Read the model definition and answer for the solid it produces. Units are mm, in the model's axes. A direction names the side the tool comes from. Coordinates: 2 decimals unless noted, no trailing zeros. Write each loop counter-clockwise with the first axis right and the second up, starting at its lowest first coordinate (ties: lowest second). Pieces come first, ordered by that corner, then holes. Notation, with made-up numbers: (-3, 83.5) -> (20, 83.5) arc R20 ccw to (20, 107.5) -> close; hole circle Ø9 at (-18, 63.5). An arc over 180 degrees is marked (long way). Answer as a JSON object with one key per item and string values. Group by question number.
(1) Find section B-B (z = -11.5). Give the vertices of the cut face in (x, y), then the cut area to 3 significant figures.
(2) Find section C-C (x = 4). Give the vertices of the cut face in (y, z).
(3) Straight lines are drawn through the part: L1, parallel to Z at x = 8.75, y = 9.25; L2, parallel to Y at x = 1, z = 0; L3, parallel to X at y = 4.25, z = -11.5. For each, find the intervals that lie inside material, in ascending order.
(4) For a pull along Y with two mould halves and no side action, classify faces 1 (the face through (4, 4.2, 0)), 2 (the face through (9.699, 11.677, 5.714)), 3 (the face through (-5.74, 13.94, 5.71)), 4 (the face through (-3, 5, 0)) as +Y half, -Y half, draft (parallel to the pull), parting line (faces both ways), or undercut.
(5) Flat-ended cylindrical pins translate along their axes: P1, Ø1, axis at x = 3.5, y = 14.5, coming from the -Z side; P2, Ø1.8, axis at x = -4.5, z = 0, coming from the -Y side; P3, Ø0.5, axis at y = 3.5, z = 4, coming from the -X side. Find the tip coordinate at first contact, or state that the pin passes through.
(6) Find section A-A (x = 0). Give the vertices of the cut face in (y, z), then the cut area to 3 significant figures.
(7) Which of the six approach directions +Z, -Z, +X, -X, +Y, -Y give full straight-line access (tool end or side, diameter ignored) to faces 5 (the face through (-1.2, 3.1, 9.9)), 6 (the face through (-4, 4.2, 0)), 7 (the face through (0, 6.1, 14))?
(8) Find section D-D (z = -8). Give the vertices of the cut face in (x, y).
from build123d import *

# Parameters (mm, degrees)
BOSS_EXTRUDE1_DEPTH     = 16
SKETCH2_W               = 20
SKETCH2_H               = 11.997864578
BOSS_EXTRUDE2_DEPTH     = 12
CHAMFER1_SIZE           = 8
FILLET1_R               = 1
CUT_EXTRUDE1_DEPTH      = 27.145936587
CUT_EXTRUDE1_DEPTH_BACK = 27.145936587
SKETCH3_R               = 4
SKETCH4_R               = 2
CUT_EXTRUDE2_DEPTH      = 23.36067982


with BuildPart() as part:
    # Sketch1 → Boss-Extrude1 (new, symmetric)
    with BuildSketch(Plane.XY):
        Polygon((-3, 6.1), (3, 6.1), (3, 4.2), (5.3, 4.2), (5.3, 2.58), (2.8, 0), (-2.8, 0), (-5.3, 2.58), (-5.3, 4.2), (-3, 4.2), align=None)
    extrude(amount=BOSS_EXTRUDE1_DEPTH, both=True)

    # Sketch2 → Boss-Extrude2 (add)
    with BuildSketch(Plane(origin=(0, 6.1, 0), x_dir=(1, 0, 0), z_dir=(0, 1, 0))):
        Rectangle(SKETCH2_W, SKETCH2_H)
    extrude(amount=BOSS_EXTRUDE2_DEPTH)

    # Chamfer1
    chamfer1_edges = [part.edges().sort_by_distance(p)[0] for p in [
        (-10, 18.1, 0),
    ]]
    chamfer(chamfer1_edges, length=CHAMFER1_SIZE)

    # Fillet1
    fillet1_edges = [part.edges().sort_by_distance(p)[0] for p in [
        (0, 6.1, -5.998932289),
        (0, 6.1, 5.998932289),
        (-10, 6.1, 0),
        (-10, 8.1, 5.998932289),
        (-10, 8.1, -5.998932289),
        (10, 6.1, 0),
        (-6, 14.1, 5.998932289),
        (-6, 14.1, -5.998932289),
        (4, 18.1, -5.998932289),
        (4, 18.1, 5.998932289),
        (10, 12.1, -5.998932289),
        (10, 18.1, 0),
        (10, 12.1, 5.998932289),
        (-2, 18.1, 0),
        (-10, 10.1, 0),
    ]]
    fillet(fillet1_edges, radius=FILLET1_R)

    # Sketch3 → Cut-Extrude1 (cut, two sides: drawn at the far end of the back side and taken through both)
    with BuildSketch(Plane(origin=(0, 0, 0), x_dir=(0, 0, -1), z_dir=(1, 0, 0)).offset(-CUT_EXTRUDE1_DEPTH_BACK)):
        with Locations((0, 12.1)):
            Circle(SKETCH3_R)
    extrude(amount=CUT_EXTRUDE1_DEPTH + CUT_EXTRUDE1_DEPTH_BACK, mode=Mode.SUBTRACT)

    # Sketch4 → Cut-Extrude2 (cut, through all)
    with BuildSketch(Plane(origin=(0, 6.1, 0), x_dir=(1, 0, 0), z_dir=(0, 1, 0))):
        with Locations(Location((0, 11.5, 0), (0, 0, 270))):
            Circle(SKETCH4_R)
        with Locations(Location((0, -11.5, 0), (0, 0, 270))):
            Circle(SKETCH4_R)
    extrude(amount=-CUT_EXTRUDE2_DEPTH, mode=Mode.SUBTRACT)


solid = part.part
Results below:
{
 "1": {"outline": "(-5.3, 2.58) -> (-2.8, 0) -> (-2, 0) -> (-2, 6.1) -> (-3, 6.1) -> (-3, 4.2) -> (-5.3, 4.2) -> close; (2, 0) -> (2.8, 0) -> (5.3, 2.58) -> (5.3, 4.2) -> (3, 4.2) -> (3, 6.1) -> (2, 6.1) -> close", "area": "25.1 mm2"},
 "2": {"outline": "(1.24, -16) -> (4.2, -16) -> (4.2, 16) -> (1.24, 16) -> close; (6.1, -6) -> (17.1, -6) arc R1 ccw to (18.1, -5) -> (18.1, 5) arc R1 ccw to (17.1, 6) -> (6.1, 6) -> close; hole circle Ø8 at (12.1, 0)"},
 "3": {"L1": "z = -6 to -2.81, 2.81 to 6", "L2": "y = 0 to 8.1, 16.1 to 18.1", "L3": "x = -3 to -2, 2 to 3"},
 "4": {"face 1": "undercut", "face 2": "draft", "face 3": "+Y half", "face 4": "undercut"},
 "5": {"P1": "stops at z = -6", "P2": "stops at y = 0.83", "P3": "stops at x = -5.3"},
 "6": {"outline": "(0, -16) -> (6.1, -16) -> (6.1, -13.5) -> (0, -13.5) -> close; (0, -9.5) -> (6.1, -9.5) -> (6.1, -7) arc R1 cw to (7.1, -6) -> (17.1, -6) arc R1 ccw to (18.1, -5) -> (18.1, 5) arc R1 ccw to (17.1, 6) -> (7.1, 6) arc R1 cw to (6.1, 7) -> (6.1, 9.5) -> (0, 9.5) -> close; (0, 13.5) -> (6.1, 13.5) -> (6.1, 16) -> (0, 16) -> close; hole circle Ø8 at (12.1, 0)", "area": "240 mm2"},
 "7": {"face 5": "+Y, -Y", "face 6": "+Z, -Z, -X", "face 7": "+Z, +X, -X, +Y"},
 "8": {"outline": "(-5.3, 2.58) -> (-2.8, 0) -> (2.8, 0) -> (5.3, 2.58) -> (5.3, 4.2) -> (3, 4.2) -> (3, 6.1) -> (-3, 6.1) -> (-3, 4.2) -> (-5.3, 4.2) -> close"}
}
